The listing builds one solid part. Answer for the finished solid, in the listing's coordinates (mm). Coordinates: 2 decimals unless noted, no trailing zeros. Order: outer loops, then holes, each group sorted by start corner. A loop starts at its lowest first (then second) coordinate and runs counter-clockwise, first axis right, second up.
from build123d import *

# Parameters (mm, degrees)
BOSS_EXTRUDE1_DEPTH = 10
FILLET1_R           = 0.5


with BuildPart() as part:
    # Sketch1 → Boss-Extrude1 (new body)
    with BuildSketch(Plane(origin=(0, 0, 0), x_dir=(1, 0, 0), z_dir=(0, 1, 0))):
        Polygon((0, 0), (30, 0), (25.980762114, 15), align=None)
    extrude(amount=BOSS_EXTRUDE1_DEPTH)

    # Fillet1
    fillet1_edges = [part.edges().sort_by_distance(p)[0] for p in [
        (30, 5, 0),
        (0, 5, 0),
        (25.980762114, 5, -15),
    ]]
    fillet(fillet1_edges, radius=FILLET1_R)


solid = part.part
(1) Find section A-A on y = 2.75. Determine the outline of the cut face in (x, z), then the cut area to 3 significant figures.
(2) Given pin 1 Ø1.5 at (y, z) = (5, -9) entering from -X; pin 2 Ø1 at (y, z) = (7.5, -11) entering from +X; pin 3 Ø1 at (y, z) = (5.5, -6.5) entering from -X, each flat-ended and moving along its own axis, determine where each tip first touches the part or whether it passes through.
(3) Find section B-B on x = 14.25. Determine the outline of the cut face in (y, z), then the cut area to 3 significant figures.
(4) Find section C-C on z = -10.25. Determine the outline of the cut face in (x, y).
(5) Find the intervals of material crossed by probe 1 along Z at (x, y) = (19.25, 8.75); probe 2 along X at (y, z) = (5, -11); probe 3 along Z at (x, y) = (9, 6.5), in increasing order.
Resolved:
1. outline: (1.62, -0.93) - (25.42, -14.67) arc R0.5 ccw to (26.15, -14.37) - (29.83, -0.63) arc R0.5 ccw to (29.35, 0) - (1.87, 0) arc R0.5 ccw to start
1. area: 224 mm2
2. pin 1: stops at x = 14.29
2. pin 2: stops at x = 27.19
2. pin 3: stops at x = 10.39
3. outline: (0, -8.23) - (10, -8.23) - (10, 0) - (0, 0) - close
3. area: 82.3 mm2
4. outline: (17.75, 0) - (27.25, 0) - (27.25, 10) - (17.75, 10) - close
5. probe 1: z = -11.11 to 0
5. probe 2: x = 19.05 to 27.05
5. probe 3: z = -5.2 to 0
